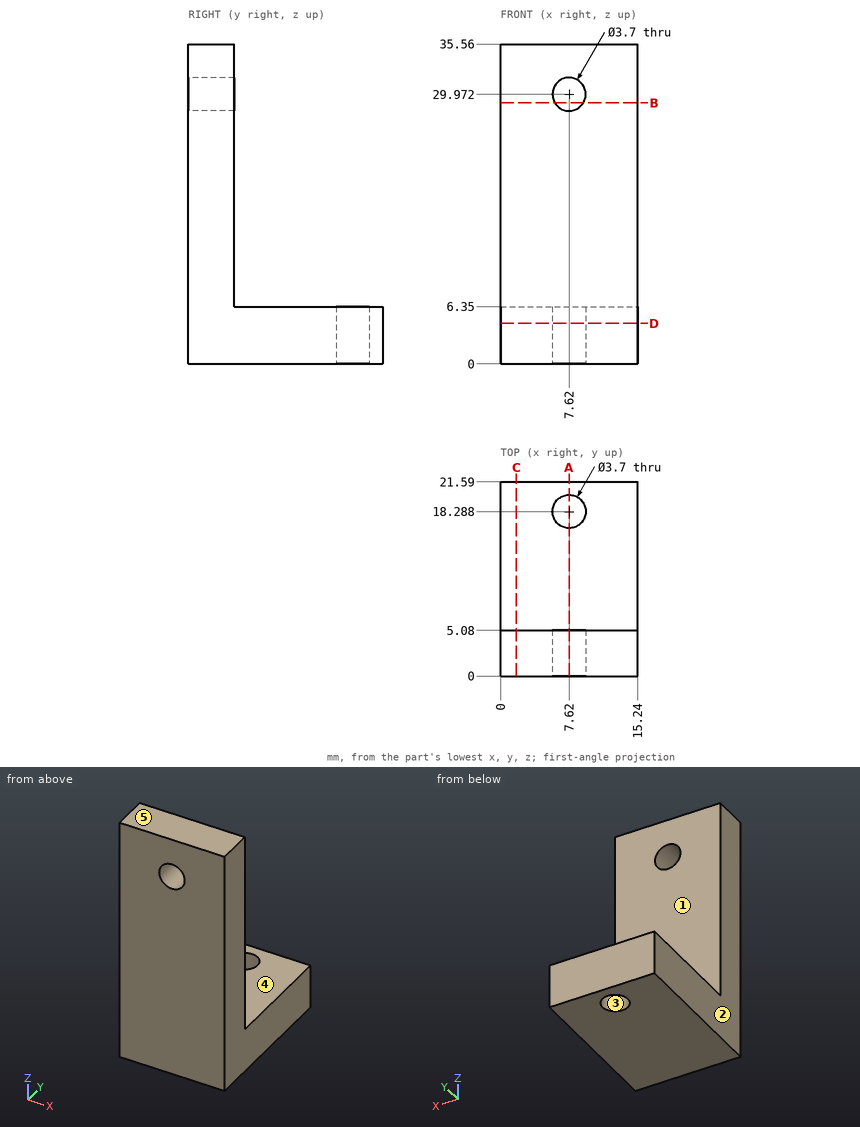
Job drawing, mm, ordinate dimensions from the low corner. One solid piece. A direction names the side the tool comes from. Coordinates: 2 decimals unless noted, no trailing zeros. Loops run counter-clockwise (first coordinate to the right, second up) from the corner with the lowest first, then second, coordinate; pieces in that order, holes last. Notation, with made-up numbers: (23, 88.25) - (51, 88.25) arc R18 ccw to (51, 105.25) - close; hole circle Ø3 at (34.5, -29). An arc over 180 degrees is marked (long way). Write item = value, one per line. Start each with the question number.
Q1. Cut at D-D, the plane z = 4.5. List the corners of the cut face in (x, y), then the cut area to 3 significant figures.
Q2. Drill centre lines: L1, parallel to Y at x = 7.62, z = 3.5; L2, parallel to Z at x = 7.62, y = 3.7; L3, parallel to Z at x = 10, y = 8.5. Where is each one in solid material? Low to high.
Q3. Cut at A-A, the plane x = 7.62. List the corners of the cut face in (y, z).
Q4. Cut at C-C, the plane x = 1.75. List the corners of the cut face in (y, z).
Q5. Which spindle directions (+Z, -Z, +X, -X, +Y, -Y) get a long thin tool onto all of the face, cutting with end or side? Do the marked faces 4 and 5. Say none if no direction does.
Q6. Pull direction Y, two halves, no side cores. Call the marked faces 1, 2 and 3: pulls with the +Y half, pulls with the -Y half, needs draft (parallel to the pull), parting line crosses it, or undercut.
Q7. Flat gauge pins, fed straight in: pin 1 Ø12 at (y, z) = (15, 10) entering from +X; pin 2 Ø7.5 at (x, z) = (10.5, 16.5) entering from +Y. Where does each tip first touch, or does it go through?
Q8. Cut at B-B, the plane z = 29. List the corners of the cut face in (x, y), then the cut area to 3 significant figures.
Computed:
q1.outline = (0, 0) - (15.24, 0) - (15.24, 21.59) - (0, 21.59) - close; hole circle Ø3.7 at (7.62, 18.29)
q1.area = 318 mm²
q2.L1 = 0 to 16.44, 20.14 to 21.59
q2.L2 = 0 to 28.12, 31.82 to 35.56
q2.L3 = 0 to 6.35
q3.outline = (0, 0) - (16.44, 0) - (16.44, 6.35) - (5.08, 6.35) - (5.08, 28.12) - (0, 28.12) - close; (0, 31.82) - (5.08, 31.82) - (5.08, 35.56) - (0, 35.56) - close; (20.14, 0) - (21.59, 0) - (21.59, 6.35) - (20.14, 6.35) - close
q4.outline = (0, 0) - (21.59, 0) - (21.59, 6.35) - (5.08, 6.35) - (5.08, 35.56) - (0, 35.56) - close
q5.face_4 = +Z, +X, -X, +Y
q5.face_5 = +Z, +X, -X, +Y, -Y
q6.face_1 = pulls with the +Y half
q6.face_2 = needs draft
q6.face_3 = undercut
q7.pin_1 = 15.24
q7.pin_2 = 5.08
q8.outline = (0, 0) - (6.05, 0) - (6.05, 5.08) - (0, 5.08) - close; (9.19, 0) - (15.24, 0) - (15.24, 5.08) - (9.19, 5.08) - close
q8.area = 61.4 mm²
